```python
from build123d import *

# Parameters (mm, degrees)
F0_R     = 3.1
F1_DEPTH = 10
F2_DEPTH = 1.5
F3_W     = 15
F3_H     = 2
F4_DEPTH = 11.501


# Not quite as in the source:
# - a feature names something its author has since deleted; it is built from what else it names


with BuildPart() as f1:
    # F0 (on Top) → F1 (new body, symmetric)
    with BuildSketch(Plane.XY):
        Circle(F0_R)
    extrude(amount=F1_DEPTH, both=True)

    # F0 (on Top) → F2 (join, symmetric)
    with BuildSketch(Plane.XY):
        with BuildLine():
            ThreePointArc((1.2599617485, -9.9203072731), (7.5033198481, -6.6106120184), (10, 0))
            ThreePointArc((10, 0), (7.503319686, 6.6106122023), (1.2599612621, 9.9203073349))
            ThreePointArc((1.2599612621, 9.9203073349), (-10, -2.451e-07), (1.2599617485, -9.9203072731))
        make_face()
        Circle(F0_R, mode=Mode.SUBTRACT)
        with BuildLine():
            ThreePointArc((1.2599612621, 9.9203073349), (7.503319686, 6.6106122023), (10, 0))
            ThreePointArc((10, 0), (7.5033198481, -6.6106120184), (1.2599617485, -9.9203072731))
            Line((1.2599617485, -9.9203072731), (40, -5))
            Line((40, -5), (40, 5))
            Line((40, 5), (1.2599612621, 9.9203073349))
        make_face()
    extrude(amount=F2_DEPTH, both=True)

    # F3 (on face) → F4 (cut, through all)
    with BuildSketch(Plane.XY.offset(1.5)):
        with Locations((32.5, 0)):
            Rectangle(F3_W, F3_H)
    extrude(amount=-F4_DEPTH, mode=Mode.SUBTRACT)


solid = f1.part
```
CAD build for the part. Positions are in the model's coordinates, mm. A direction names the side the tool comes from. Give positions to 0.01 mm unless a question says otherwise; leave off trailing zeros. Write each loop counter-clockwise with the first axis right and the second up, starting at its lowest first coordinate (ties: lowest second). Pieces come first, ordered by that corner, then holes. Notation, with made-up numbers: M 10.25,-32.5 L 69.25,-32.5 A19 ccw 69.25,-15.5 Z; hole C 16.5,11 d4. An arc over 180 degrees is marked long. Return JSON: item names as keys, results as strings. Group by question number.
(1) 3-axis set-ups, long thin cutter, end or side, ignore diameter. For faces 5 (the face through (32, 1, 0)), 6 (the face through (1.43, -2.75, -5.69)), 7 (the face through (0, 0, 10)): which of +Z, -Z, +X, -X, +Y, -Y reach the whole face in a straight line?
(2) Band-saw the part on D-D (y = 6.5). Give the cut face in (x, z).
(3) Flat gauge pins, fed straight in: pin 1 Ø1.5 at (x, z) = (32.5, 3) entering from -Y; pin 2 Ø6 at (x, z) = (-4.5, 1) entering from +Y; pin 3 Ø6 at (x, z) = (3, 5) entering from -Y; pin 4 Ø3 at (x, y) = (-2, 6.5) entering from +Z. Where does each tip first touch, or does it go through?
(4) Mould opens along Y. For faces 1 (the face through (1.43, -2.75, 5.81)), 2 (the face through (40, -3, 0)), 3 (the face through (32, -1, 0)), 4 (the face through (25, 0, 0)) say: pulls with the +Y half, pulls with the -Y half, needs draft (parallel to the pull), parting line crosses it, or undercut.
(5) Band-saw the part on B-B (x = 0). Give the cut face in (y, z).
(6) Drill centre lines: L1, parallel to Z at x = 30, y = -1.5; L2, parallel to X at y = 0.5, z = -5.25; L3, parallel to Y at x = 17, z = -0.75. Where is each one in solid material? Low to high. Write a range as [from, to].
(7) Band-saw the part on A-A (y = 0). Give the cut face in (x, z), and give its area (3 significant figures).
(8) Band-saw the part on C-C (z = -2.5). Give the cut face in (x, y).
Entries:
{
 "1": {"face 5": "+Z, -Z, +X", "face 6": "-Z", "face 7": "+Z, +X, -X, +Y, -Y"},
 "2": {"outline": "M -7.6,-1.5 L 28.19,-1.5 L 28.19,1.5 L -7.6,1.5 Z"},
 "3": {"pin 1": "passes through", "pin 2": "stops at y = 9.89", "pin 3": "stops at y = -3.1", "pin 4": "stops at z = 1.5"},
 "4": {"face 1": "parting line crosses it", "face 2": "needs draft", "face 3": "undercut", "face 4": "undercut"},
 "5": {"outline": "M -10,-1.5 L -3.1,-1.5 L -3.1,-10 L 3.1,-10 L 3.1,-1.5 L 10,-1.5 L 10,1.5 L 3.1,1.5 L 3.1,10 L -3.1,10 L -3.1,1.5 L -10,1.5 Z"},
 "6": {"L1": "z = [-1.5, 1.5]", "L2": "x = [-3.06, 3.06]", "L3": "y = [-7.92, 7.92]"},
 "7": {"outline": "M -10,-1.5 L -3.1,-1.5 L -3.1,-10 L 3.1,-10 L 3.1,-1.5 L 25,-1.5 L 25,1.5 L 3.1,1.5 L 3.1,10 L -3.1,10 L -3.1,1.5 L -10,1.5 Z", "area": "210 mm^2"},
 "8": {"outline": "C 0,0 d6.2"}
}
